Source: CAD feature listing. Evaluate the final solid. Frame: model axes, mm. A direction names the side the tool comes from. Round coordinates to 2 decimals unless told otherwise and drop trailing zeros. Write each loop counter-clockwise with the first axis right and the second up, starting at its lowest first coordinate (ties: lowest second). Pieces come first, ordered by that corner, then holes. Notation, with made-up numbers: (2.25, 20.5) - (46.25, 20.5) arc R11 ccw to (46.25, 36.5) - close; hole circle Ø7 at (65, 10.25). An arc over 180 degrees is marked (long way). Write item = value, one per line. Start each with the question number.
```python
from build123d import *

# Parameters (mm, degrees)
F2_R     = 19
F3_DEPTH = 3
F4_R     = 2.99999


# Not quite as in the source:
# - a fillet or chamfer is up to 0.001 mm smaller than in the source, because OpenCascade refuses the exact size


with BuildPart() as f1:
    # F0 (on Top) → F1 (revolve)
    with BuildSketch(Plane.XY):
        with BuildLine():
            Line((0, 0), (-20, 0))
            ThreePointArc((-20, 0), (-15.7989821534, -12.2634482474), (-4.9607837082, -19.375))
            ThreePointArc((-4.9607837082, -19.375), (-3.75, -23.3071891388), (0, -25))
            Line((0, -25), (0, -20))
            Line((0, -20), (0, 0))
        make_face()
    revolve(axis=Axis((0, -10, 0), (0, -1, 0)))

    # F2 (on Front) → F3 (join)
    with BuildSketch(Plane.XZ):
        Circle(F2_R)
    extrude(amount=-F3_DEPTH)

    # F4 (radius 3 in the source; OpenCascade refuses exactly that, so slightly less here)
    f4_edges = [f1.edges().sort_by_distance(p)[0] for p in [
        (-19, 3, 0),
    ]]
    fillet(f4_edges, radius=F4_R)


solid = f1.part
```
(1) Reachability of faces 1 (the flat face through (0, 3, 0)), 2 (the flat face through (18, 0, 7)) from +Z, -Z, +X, -X, +Y, -Y: full face, straight path, thin tool, end or side. Return the list, or none.
(2) Section C-C (y = -17.25). Return the cut outline in (x, z), plus the area to 3 significant figures.
(3) Contact query for flat-ended pins moving along their axis: P1, Ø2, axis at x = -8, y = -4, coming from the +Z side; P2, Ø4, axis at x = -9, y = -14, coming from the -Z side; P3, Ø4, axis at x = -15.5, z = -13.5, coming from the -Y side. Output: stop coordinate, or through.
(4) Section D-D (y = -3.5). Return the cut outline in (x, z), plus the area to 3 significant figures.
(5) Ray query, L1, parallel to Z at x = 4, y = -4.75; L2, parallel to Y at x = 10, z = -4; L3, parallel to X at y = -6, z = 15. Return the intervals inside material, ascending. Write a range as from..to.
Solution:
q1.face_1 = +Z, -Z, +X, -X, +Y
q1.face_2 = +Y
q2.outline = circle Ø20.24 at (0, 0)
q2.area = 322 mm^2
q3.P1 = 18.35
q3.P2 = -13.62
q3.P3 = -7.46
q4.outline = circle Ø39.38 at (0, 0)
q4.area = 1,220 mm^2
q5.L1 = -19.01..19.01
q5.L2 = -16.85..3
q5.L3 = -11.79..11.79
